from build123d import *

# Parameters (mm, degrees)
CYLINDER050_R           = 1.7
CYLINDER050_DEPTH       = 20
CYLINDER050_PITCH_ANGLE = 90
CYLINDER049_R           = 1.7
CYLINDER049_DEPTH       = 20
CYLINDER049_PITCH_ANGLE = 90
CYLINDER051_R           = 1.7
CYLINDER051_DEPTH       = 20
CYLINDER051_PITCH_ANGLE = 90
CYLINDER047_R           = 1.7
CYLINDER047_DEPTH       = 20
CYLINDER047_PITCH_ANGLE = 90
CYLINDER046_R           = 1.7
CYLINDER046_DEPTH       = 20
CYLINDER046_PITCH_ANGLE = 90
CYLINDER048_R           = 1.7
CYLINDER048_DEPTH       = 20
CYLINDER048_PITCH_ANGLE = 90
SKETCH023_R             = 1.7
PAD021_DEPTH            = 20
SKETCH024_R             = 1.7
PAD022_DEPTH            = 20
CYLINDER001_R           = 5
CYLINDER001_DEPTH       = 50
CYLINDER_R              = 5
CYLINDER_DEPTH          = 50
SKETCH002_W             = 400
SKETCH002_H             = 300
PAD002_DEPTH            = 10


with BuildPart() as cylinder050:
    # Cylinder050 → Cylinder050 (new body)
    with BuildSketch(Plane.XY):
        Circle(CYLINDER050_R)
    extrude(amount=CYLINDER050_DEPTH)


with BuildPart() as cylinder050_1:
    # Cylinder050 pitch: moved
    add(cylinder050.part.rotate(Axis((0, 0, 0), (0, 1, 0)), CYLINDER050_PITCH_ANGLE))


with BuildPart() as cylinder050_2:
    # Cylinder050 placement: moved
    add(cylinder050_1.part.moved(Location((-220, 120, -5))))


with BuildPart() as cylinder049:
    # Cylinder049 → Cylinder049 (new body)
    with BuildSketch(Plane.XY):
        Circle(CYLINDER049_R)
    extrude(amount=CYLINDER049_DEPTH)


with BuildPart() as cylinder049_1:
    # Cylinder049 pitch: moved
    add(cylinder049.part.rotate(Axis((0, 0, 0), (0, 1, 0)), CYLINDER049_PITCH_ANGLE))


with BuildPart() as cylinder049_2:
    # Cylinder049 placement: moved
    add(cylinder049_1.part.moved(Location((-220, -90, -5))))


with BuildPart() as fusion016:
    # Cylinder051 → Cylinder051 (new body)
    with BuildSketch(Plane.XY):
        Circle(CYLINDER051_R)
    extrude(amount=CYLINDER051_DEPTH)


with BuildPart() as fusion016_1:
    # Cylinder051 pitch: moved
    add(fusion016.part.rotate(Axis((0, 0, 0), (0, 1, 0)), CYLINDER051_PITCH_ANGLE))


with BuildPart() as fusion016_2:
    # Cylinder051 placement: moved
    add(fusion016_1.part.moved(Location((-220, 15, -5))))

    # Fusion016: union Cylinder050, Cylinder049
    add(cylinder050_2.part)
    add(cylinder049_2.part)


with BuildPart() as fusion016_3:
    # Fusion016 placement: moved
    add(fusion016_2.part.moved(Location((415, -5, 0))))


with BuildPart() as cylinder047:
    # Cylinder047 → Cylinder047 (new body)
    with BuildSketch(Plane.XY):
        Circle(CYLINDER047_R)
    extrude(amount=CYLINDER047_DEPTH)


with BuildPart() as cylinder047_1:
    # Cylinder047 pitch: moved
    add(cylinder047.part.rotate(Axis((0, 0, 0), (0, 1, 0)), CYLINDER047_PITCH_ANGLE))


with BuildPart() as cylinder047_2:
    # Cylinder047 placement: moved
    add(cylinder047_1.part.moved(Location((-220, 120, -5))))


with BuildPart() as cylinder046:
    # Cylinder046 → Cylinder046 (new body)
    with BuildSketch(Plane.XY):
        Circle(CYLINDER046_R)
    extrude(amount=CYLINDER046_DEPTH)


with BuildPart() as cylinder046_1:
    # Cylinder046 pitch: moved
    add(cylinder046.part.rotate(Axis((0, 0, 0), (0, 1, 0)), CYLINDER046_PITCH_ANGLE))


with BuildPart() as cylinder046_2:
    # Cylinder046 placement: moved
    add(cylinder046_1.part.moved(Location((-220, -90, -5))))


with BuildPart() as fusion015:
    # Cylinder048 → Cylinder048 (new body)
    with BuildSketch(Plane.XY):
        Circle(CYLINDER048_R)
    extrude(amount=CYLINDER048_DEPTH)


with BuildPart() as fusion015_1:
    # Cylinder048 pitch: moved
    add(fusion015.part.rotate(Axis((0, 0, 0), (0, 1, 0)), CYLINDER048_PITCH_ANGLE))


with BuildPart() as fusion015_2:
    # Cylinder048 placement: moved
    add(fusion015_1.part.moved(Location((-220, 15, -5))))

    # Fusion015: union Cylinder047, Cylinder046
    add(cylinder047_2.part)
    add(cylinder046_2.part)


with BuildPart() as fusion015_3:
    # Fusion015 placement: moved
    add(fusion015_2.part.moved(Location((5, -5, 0))))


with BuildPart() as pad021:
    # Sketch023 → Pad021 (new body)
    with BuildSketch(Plane.XZ.offset(135)):
        with Locations((-150, -5)):
            Circle(SKETCH023_R)
        with Locations((0, -5)):
            Circle(SKETCH023_R)
        with Locations((150, -5)):
            Circle(SKETCH023_R)
    extrude(amount=PAD021_DEPTH)


with BuildPart() as fusion017:
    # Sketch024 → Pad022 (new body)
    with BuildSketch(Plane.XZ.offset(-175)):
        with Locations((-150, -5)):
            Circle(SKETCH024_R)
        with Locations((0, -5)):
            Circle(SKETCH024_R)
        with Locations((150, -5)):
            Circle(SKETCH024_R)
    extrude(amount=PAD022_DEPTH)

    # Fusion017: union Fusion016, Fusion015, Pad021
    add(fusion016_3.part)
    add(fusion015_3.part)
    add(pad021.part)


with BuildPart() as cylinder001:
    # Cylinder001 → Cylinder001 (new body)
    with BuildSketch(Plane(origin=(-155, -66, -30), x_dir=(1, 0, 0), z_dir=(0, 0, 1))):
        Circle(CYLINDER001_R)
    extrude(amount=CYLINDER001_DEPTH)


with BuildPart() as fusion018:
    # Cylinder → Cylinder (new body)
    with BuildSketch(Plane(origin=(155, -66, -25), x_dir=(1, 0, 0), z_dir=(0, 0, 1))):
        Circle(CYLINDER_R)
    extrude(amount=CYLINDER_DEPTH)

    # Fusion018: union Cylinder001
    add(cylinder001.part)


with BuildPart() as cut018:
    # Sketch002 → Pad002 (new body)
    with BuildSketch(Plane(origin=(0, 0, -10), x_dir=(1, 0, 0), z_dir=(0, 0, -1))):
        with Locations((0, -10)):
            Rectangle(SKETCH002_W, SKETCH002_H)
    extrude(amount=-PAD002_DEPTH)

    # Cut: cut Fusion018
    add(fusion018.part, mode=Mode.SUBTRACT)

    # Cut018: cut Fusion017
    add(fusion017.part, mode=Mode.SUBTRACT)


solid = cut018.part
Read the model definition and answer for the solid it produces. Units are mm, in the model's axes. Coordinates: 2 decimals unless noted, no trailing zeros. Loops run counter-clockwise (first coordinate to the right, second up) from the corner with the lowest first, then second, coordinate; pieces in that order, holes last. Notation, with made-up numbers: (52, 44) -> (69, 44) arc R28 cw to (69, 71) -> close; hole circle Ø10 at (67, 48.5). An arc over 180 degrees is marked (long way). Answer in a Markdown table with one row per item.
Item 1: Each of these flat-tipped pins is pushed along its axis until it touches: P1, Ø2.5, axis at x = 0, z = -5, coming from the -Y side; P2, Ø1, axis at y = 10.5, z = -5.5, coming from the +X side; P3, Ø3, axis at x = 0, z = -5, coming from the +Y side. Where does it stop, or does it pass through?
Returned:
| item | result |
|---|---|
| P1 | stops at y = -135 |
| P2 | stops at x = 195 |
| P3 | stops at y = 155 |
Item 2: A cutting plane is placed at A-A on y = -66. Determine the outline of the cut face in (x, z).
Returned:
| item | result |
|---|---|
| outline | (-200, -10) -> (-160, -10) -> (-160, 0) -> (-200, 0) -> close; (-150, -10) -> (150, -10) -> (150, 0) -> (-150, 0) -> close; (160, -10) -> (200, -10) -> (200, 0) -> (160, 0) -> close |
Item 3: For a pull along X with two mould halves and no side action, classify faces 1 (the cylindrical face through (-159, -63, -5)), 2 (the flat face through (-3, 8, 0)), 3 (the flat face through (-200, 12, -5)), 4 (the cylindrical face through (151, -63, -5)) as released by +X, released by -X, zero draft, split by the parting line, or undercut.
Returned:
| item | result |
|---|---|
| face 1 | undercut |
| face 2 | zero draft |
| face 3 | released by -X |
| face 4 | undercut |
Item 4: Straight lines are drawn through the part: line 1 along X through (y, z) = (158.3, -5); line 2 along Y through (x, z) = (198.35, -5); line 3 along Z through (x, y) = (0, -138). For each, find the intervals that lie inside material, in ascending order. Write a range as [from, to].
Returned:
| item | result |
|---|---|
| line 1 | x = [-200, -151.7], [-148.3, -1.7], [1.7, 148.3], [151.7, 200] |
| line 2 | y = [-140, -96.7], [-93.3, 8.3], [11.7, 113.3], [116.7, 160] |
| line 3 | z = [-10, -6.7], [-3.3, 0] |
